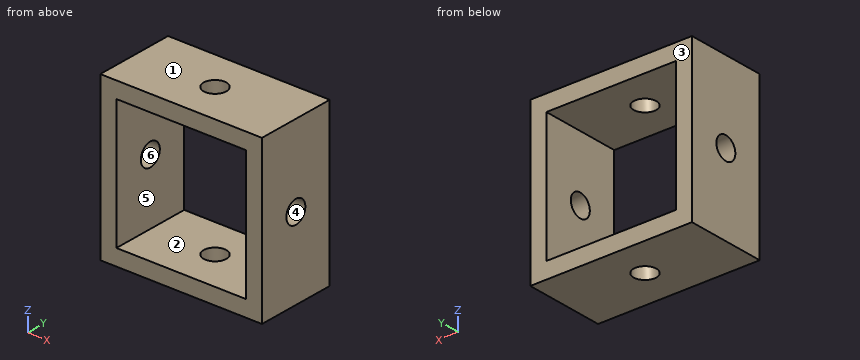
from build123d import *

# Parameters (mm, degrees)
SKETCH1_W           = 50
SKETCH1_H           = 50
SKETCH1_W_2         = 40
SKETCH1_H_2         = 40
BOSS_EXTRUDE1_DEPTH = 25
SKETCH2_R           = 3.5
CUT_EXTRUDE1_DEPTH  = 55
SKETCH3_R           = 3.5
CUT_EXTRUDE2_DEPTH  = 55


with BuildPart() as part:
    # Sketch1 → Boss-Extrude1 (new body)
    with BuildSketch(Plane(origin=(0, 0, 0), x_dir=(1, 0, 0), z_dir=(0, 1, 0))):
        Rectangle(SKETCH1_W, SKETCH1_H)
        Rectangle(SKETCH1_W_2, SKETCH1_H_2, mode=Mode.SUBTRACT)
    extrude(amount=BOSS_EXTRUDE1_DEPTH)

    # Sketch2 → Cut-Extrude1 (cut)
    with BuildSketch(Plane(origin=(25, 0, 0), x_dir=(0, 0, -1), z_dir=(1, 0, 0))):
        with Locations((0, 12.5)):
            Circle(SKETCH2_R)
    extrude(amount=-CUT_EXTRUDE1_DEPTH, mode=Mode.SUBTRACT)

    # Sketch3 → Cut-Extrude2 (cut)
    with BuildSketch(Plane.XY.offset(25)):
        with Locations((0, 12.5)):
            Circle(SKETCH3_R)
    extrude(amount=-CUT_EXTRUDE2_DEPTH, mode=Mode.SUBTRACT)


solid = part.part
Work out the finished part from the listing and answer in its coordinate system (mm). Face numbers are marked on the shaded views. A direction names the side the tool comes from. Give positions to 0.01 mm unless a question says otherwise; leave off trailing zeros. Loops run counter-clockwise (first coordinate to the right, second up) from the corner with the lowest first, then second, coordinate; pieces in that order, holes last. Notation, with made-up numbers: M -35,-32 L 16,-32 A8 cw 16,-27 Z; hole C 17,15 d6. An arc over 180 degrees is marked long. Use CSV: the item, a comma, the result in double quotes.
1) Given P1, Ø6.5, axis at x = 0, y = 12.5, coming from the -Z side, flat-ended and moving along its own axis, determine where the tip first touches the part or whether it passes through.
Answer:
P1,"through"
2) Find section C-C on y = 12.5. Write down the section's boundary in (x, z).
Answer:
outline,"M -25,-25 L -3.5,-25 L -3.5,-20 L -20,-20 L -20,-3.5 L -25,-3.5 Z; M -25,3.5 L -20,3.5 L -20,20 L -3.5,20 L -3.5,25 L -25,25 Z; M 3.5,-25 L 25,-25 L 25,-3.5 L 20,-3.5 L 20,-20 L 3.5,-20 Z; M 3.5,20 L 20,20 L 20,3.5 L 25,3.5 L 25,25 L 3.5,25 Z"
3) Find section B-B on y = 5. Write down the section's boundary in (x, z), plus the area to 3 significant figures.
Answer:
outline,"M -25,-25 L 25,-25 L 25,25 L -25,25 Z; hole M -20,-20 L 20,-20 L 20,20 L -20,20 Z"
area,"900 mm^2"
4) Find section D-D on x = -14. Write down the section's boundary in (y, z).
Answer:
outline,"M 0,-25 L 25,-25 L 25,-20 L 0,-20 Z; M 0,20 L 25,20 L 25,25 L 0,25 Z"
5) Find section A-A on z = 5. Write down the section's boundary in (x, y).
Answer:
outline,"M -25,0 L -20,0 L -20,25 L -25,25 Z; M 20,0 L 25,0 L 25,25 L 20,25 Z"
6) Determine the mould class of the marked faces 3, 4, 5 and 6 for opening direction Y: released by +Y, released by -Y, zero draft, split by the parting line, or undercut.
Answer:
face 3,"released by +Y"
face 4,"undercut"
face 5,"zero draft"
face 6,"undercut"
7) Which of the six approach directions +Z, -Z, +X, -X, +Y, -Y give full straight-line access (tool end or side, diameter ignored) to the marked faces 1 and 2?
Answer:
face 1,"+Z, +X, -X, +Y, -Y"
face 2,"+Y, -Y"
8) Consider L1, parallel to Y at x = 0, z = 21; L2, parallel to X at y = 6.5, z = -4.5. Determine where each line is inside the solid, lowest interval first.
Answer:
L1,"0 to 9, 16 to 25"
L2,"-25 to -20, 20 to 25"
